The listing builds one solid part. Answer for the finished solid, in the listing's coordinates (mm). A direction names the side the tool comes from. Round coordinates to 2 decimals unless told otherwise and drop trailing zeros. Write each loop counter-clockwise with the first axis right and the second up, starting at its lowest first coordinate (ties: lowest second). Pieces come first, ordered by that corner, then holes. Notation, with made-up numbers: (41, 89.25) -> (90, 89.25) arc R26 ccw to (90, 125.25) -> close; hole circle Ø8 at (22, -38). An arc over 180 degrees is marked (long way). Write each question's results on one line, items separated by ' | '. Start each with the question number.
Autodesk Inventor part; units mm, degrees
ref_plane "YZ Plane" through (0, 0, 0) normal (1, 0, 0) x (0, 1, 0)
ref_plane "XZ Plane" through (0, 0, 0) normal (0, 1, 0) x (-1, 0, 0)
ref_plane "XY Plane" through (0, 0, 0) normal (0, 0, 1) x (1, 0, 0)
sketch "Sketch1" plane through (0, 0, 0) normal (0, 0, 1) x (1, 0, 0)
  circle A0 centre (0, 0) radius 15
  dimension "d0" = 30
extrude "Extrusion1" add sketch "Sketch1" along normal blind 53
sketch "Sketch2" plane through (0, 0, 53) normal (0, 0, 1) x (1, 0, 0)
  circle A0 centre (0, 0) radius 12.5
  dimension "d3" = 25
extrude "Extrusion2" add sketch "Sketch2" along normal blind 5
thread "Thread1"
sketch "Sketch3" plane through (0, 0, 0) normal (0, 0, -1) x (-1, 0, 0)
  circle A0 centre (0, 0) radius 6.5
  dimension "d8" = 13
extrude "Extrusion3" add sketch "Sketch3" along normal blind 4.9
sketch "Sketch4" plane through (0, 0, 0) normal (0, 0, -1) x (-1, 0, 0)
  circle A0 centre (0, 0) radius 13.5
  dimension "d11" = 27
extrude "Extrusion4" add sketch "Sketch4" along normal blind 2.5
sketch "Sketch5" plane through (0, 0, -2.5) normal (0, 0, -1) x (-1, 0, 0)
  circle A0 centre (0, 0) radius 10.15
  dimension "d14" = 20.3
extrude "Extrusion5" add sketch "Sketch5" along normal blind 2.3
chamfer "Chamfer1" distance 1.5 angle 65 1 edges at (13.5, 0, -2.5) measured on face at (-13.3252, -2.1656, -1.6667)
chamfer "Chamfer2" distance 1.6 angle 65 1 edges at (10.15, 0, -4.8) measured on face at (-10.1171, -0.8167, -4.0333)
ref_plane "Work Plane1" through (0, 0, -6.9) normal (0, 0, -1) x (-1, 0, 0)
sketch "Sketch6" plane through (0, 0, 58) normal (0, 0, 1) x (1, 0, 0)
  circle A0 centre (0, 0) radius 10
  dimension "d24" = 20
extrude "Extrusion6" cut sketch "Sketch6" against normal blind 58
sketch "Sketch7" plane through (0, 0, 0) normal (0, 0, 1) x (1, 0, 0)
  circle A0 centre (0, 0) radius 8
  dimension "d27" = 16
extrude "Extrusion7" cut sketch "Sketch7" against normal blind 2
thicken "Thicken1" operation add thickness 58 both sides no extend neighbours no toward (0, 0, 1) faces at (9.159, -1.4359, 0)
thicken "Thicken2" operation add thickness 60 both sides no extend neighbours no toward (0, 0, 1) faces at (0.9456, 2.4934, -2)
properties part number "Nikon-Objektive-MUC11900_Mockup" material "Stainless Steel"
Q1. The part is cut by section C-C, the plane z = 51. Write down the section's boundary in (x, y).
Q2. For faces 1 (the flat face through (-11.18, 7.85, 0)), 2 (the flat face through (-3.4, 12.3, 53)), 3 (the cylindrical face through (-14.985, -0.66, 26.129)), determine the directions among +Z, -Z, +X, -X, +Y, -Y from which every point of the face is accessible in a straight line to the end or side of a thin tool.
Q3. Each of these flat-tipped pins is pushed along its axis until it touches: pin 1 (2 mm diameter, centred on x = 9.5, y = -6.5, fed in from -Z); pin 2 (4 mm diameter, centred on x = -11.5, z = 15.5, fed in from -Y); pin 3 (4 mm diameter, centred on y = -6.5, z = 46, fed in from +X); pin 4 (12 mm diameter, centred on x = -3, z = 47, fed in from +Y). Where does it stop, or does it pass through?
Q4. Find the intervals of material crossed by line 1 (Z direction, x = -13, y = 6); line 2 (Y direction, x = -0.5, z = 13); line 3 (X direction, y = -1.5, z = 23), in increasing order.
Q5. The part is cut by section A-A, the plane y = 0. Write down the section's boundary in (x, z).
Answers follow:
1) outline: circle Ø30 at (0, 0)
2) face 1: -Z | face 2: +Z | face 3: +Z, -Z
3) pin 1: z = -2.39 | pin 2: y = -11.61 | pin 3: x = 14.31 | pin 4: y = 15
4) line 1: 0 to 53 | line 2: -14.99 to 14.99 | line 3: -14.92 to 14.92
5) outline: (-15, 0) -> (-13.5, 0) -> (-13.5, -1) -> (-10.28, -2.5) -> (-10.15, -2.5) -> (-10.15, -3.2) -> (-6.72, -4.8) -> (-6.5, -4.8) -> (-6.5, -4.9) -> (6.5, -4.9) -> (6.5, -4.8) -> (6.72, -4.8) -> (10.15, -3.2) -> (10.15, -2.5) -> (10.28, -2.5) -> (13.5, -1) -> (13.5, 0) -> (15, 0) -> (15, 53) -> (12.5, 53) -> (12.5, 58) -> (-12.5, 58) -> (-12.5, 53) -> (-15, 53) -> close
